Drawing for the job (mm, zero at the part's lowest x, y, z). A direction names the side the tool comes from. Coordinates: 2 decimals unless noted, no trailing zeros. Order: outer loops, then holes, each group sorted by start corner. A loop starts at its lowest first (then second) coordinate and runs counter-clockwise, first axis right, second up. Notation, with made-up numbers: M 51.5,65.25 L 106.5,65.25 A11 cw 106.5,82.25 Z; hole C 59.25,61 d1. An arc over 180 degrees is marked long. Write item = value, one per line. Start each with the question number.
Q1. Drill centre lines: probe 1 along Y at (x, z) = (35, 17.5); probe 2 along X at (y, z) = (24, 3); probe 3 along Y at (x, z) = (39, 28). Where is each one in solid material? Low to high.
Q2. Pull direction Y, two halves, no side cores. Call the marked faces 1, 2, 3 and 4: released by +Y, released by -Y, zero draft, split by the parting line, or undercut.
Q3. Band-saw the part on A-A on y = 123.5. Write the cut outline in (x, z), plus the area to 3 significant figures.
Q4. Band-saw the part on D-D on z = 42. Write the cut outline in (x, y).
Q5. Pin check, flat tips, straight feed: P1, Ø12, axis at x = 54, z = 28.5, coming from the -Y side; P2, Ø5, axis at y = 127.5, z = 8, coming from the +X side; P3, Ø12, axis at x = 52.5, y = 18.5, coming from the +Z side; P4, Ø5, axis at x = 40.5, y = 16, coming from the +Z side. Stop position of each tip, or through.
Q6. 3-axis set-ups, long thin cutter, end or side, ignore diameter. For the marked faces 5, 6, 7 and 8: which of +Z, -Z, +X, -X, +Y, -Y reach the whole face in a straight line?
Q7. Band-saw the part on C-C on z = 12. Write the cut outline in (x, y).
Q8. Band-saw the part on B-B on x = 35. Write the cut outline in (y, z).
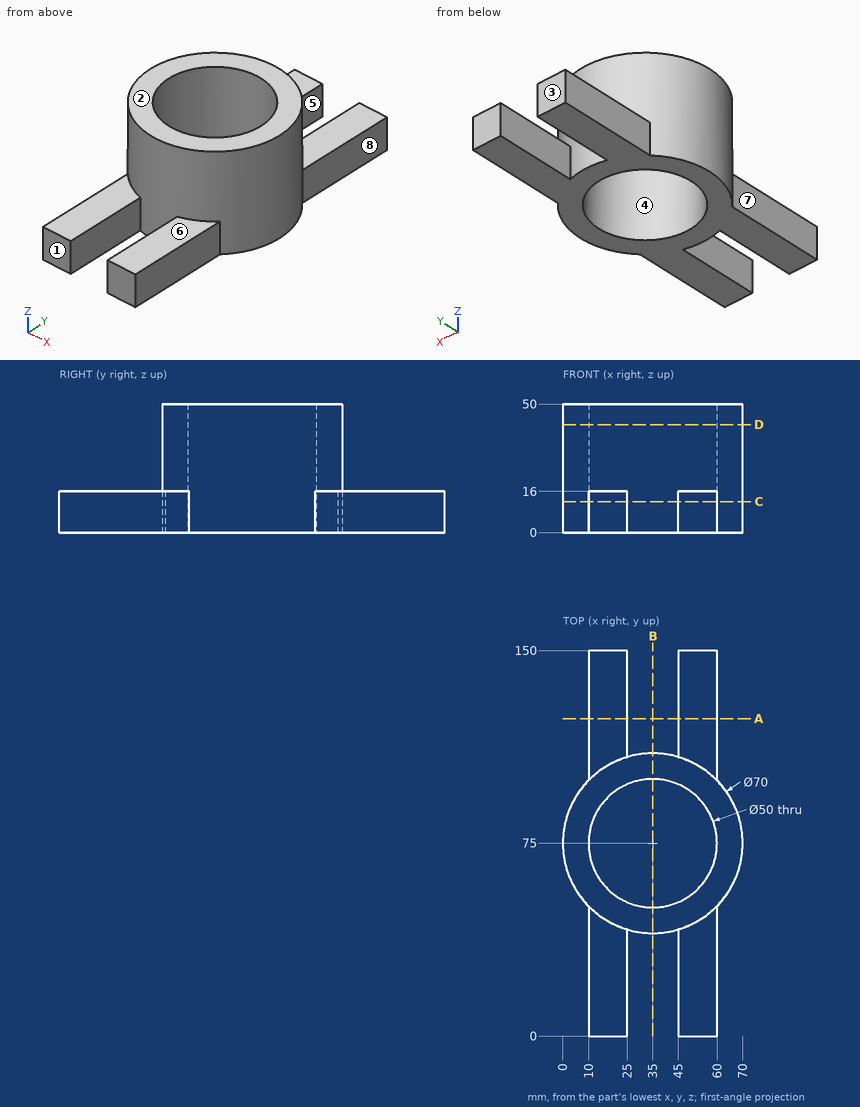
Recorded:
q1.probe_1 = 40 to 50, 100 to 110
q1.probe_2 = 10 to 25, 45 to 60
q1.probe_3 = 40.23 to 50.32, 99.68 to 109.77
q2.face_1 = released by -Y
q2.face_2 = zero draft
q2.face_3 = released by +Y
q2.face_4 = undercut
q3.outline = M 10,0 L 25,0 L 25,16 L 10,16 Z; M 45,0 L 60,0 L 60,16 L 45,16 Z
q3.area = 480 mm2
q4.outline = C 35,75 d70; hole C 35,75 d50
q5.P1 = 42.5
q5.P2 = 60
q5.P3 = 16
q5.P4 = through
q6.face_5 = +Z, -Z, +Y
q6.face_6 = +Z, +X, -Y
q6.face_7 = +Z, -Z, -X, -Y
q6.face_8 = +Z, -Z, +X, +Y
q7.outline = M 10,0 L 25,0 L 25,41.46 A35 ccw 45,41.46 L 45,0 L 60,0 L 60,50.51 A35 ccw 60,99.49 L 60,150 L 45,150 L 45,108.54 A35 ccw 25,108.54 L 25,150 L 10,150 L 10,99.49 A35 ccw 10,50.51 Z; hole C 35,75 d50
q8.outline = M 40,0 L 50,0 L 50,50 L 40,50 Z; M 100,0 L 110,0 L 110,50 L 100,50 Z
